Part model, mm, in its own coordinate system. Face numbers are marked on the shaded views. A direction names the side the tool comes from. Round coordinates to 2 decimals unless told otherwise and drop trailing zeros. Write each loop counter-clockwise with the first axis right and the second up, starting at its lowest first coordinate (ties: lowest second). Pieces come first, ordered by that corner, then holes.
from build123d import *

# Parameters (mm, degrees)
FILLET1_R          = 1.3
CHAMFER1_SIZE      = 1
CHAMFER1_SIZE2     = 0.577350269
SKETCH2_OUTSIDE_W  = 37.134
SKETCH2_OUTSIDE_H  = 37.134
CUT_EXTRUDE1_DEPTH = 8
CHAMFER2_SIZE      = 1.6


with BuildPart() as part:
    # Sketch1 → Revolve1 (revolve)
    with BuildSketch(Plane(origin=(0, 0, 0), x_dir=(0, 0, -1), z_dir=(1, 0, 0))):
        Polygon((10, 0), (10, 12), (6.5, 12), (6.5, 14), (12, 14), (12, 8), (13.5, 8), (13.5, 0), align=None)
    revolve(axis=Axis((0, 0, 0), (0, 1, 0)))

    # Fillet1
    fillet1_edges = [part.edges().sort_by_distance(p)[0] for p in [
        (0, 14, 12),
    ]]
    fillet(fillet1_edges, radius=FILLET1_R)

    # Chamfer1
    chamfer1_edges = [part.edges().sort_by_distance(p)[0] for p in [
        (0, 8, 13.5),
    ]]
    chamfer1_side = [part.faces().sort_by_distance(p)[0] for p in [
        (0, 8, 12.381837662),
    ]]
    chamfer(chamfer1_edges, length=CHAMFER1_SIZE, length2=CHAMFER1_SIZE2, reference=chamfer1_side[0])

    # Sketch2 outside → Cut-Extrude1 (cut)
    with BuildSketch(Plane.XZ):
        Rectangle(SKETCH2_OUTSIDE_W, SKETCH2_OUTSIDE_H)
        Polygon((-13.5, 0), (-6.75, -11.691342951), (6.75, -11.691342951), (13.5, 0), (6.75, 11.691342951), (-6.75, 11.691342951), align=None, mode=Mode.SUBTRACT)
    extrude(amount=-CUT_EXTRUDE1_DEPTH, mode=Mode.SUBTRACT)

    # Chamfer2
    chamfer2_edges = [part.edges().sort_by_distance(p)[0] for p in [
        (0, 0, 10),
    ]]
    chamfer(chamfer2_edges, length=CHAMFER2_SIZE)


solid = part.part
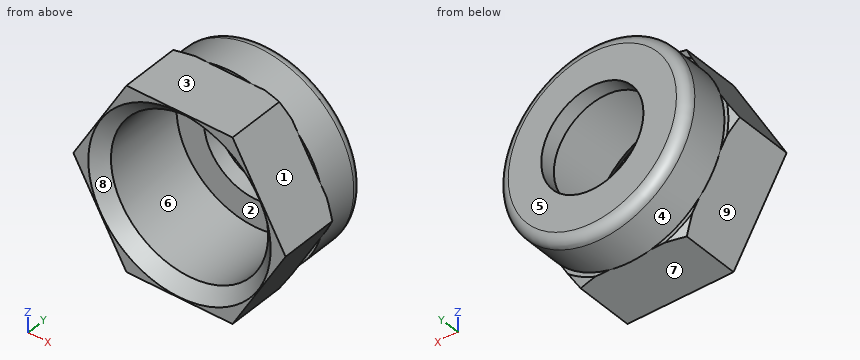
Q1. Saw through at B-B, the plane y = 6. Write the cut outline in (x, z), and give its area (3 significant figures).
Q2. Saw through at D-D, the plane y = 10. Write the cut outline in (x, z).
Q3. Drop flat-ended pins along their axis: P1, Ø0.8, axis at x = 12, z = -0.5, coming from the +Y side; P2, Ø1.5, axis at x = 8.5, y = 8, coming from the +Z side; P3, Ø1, axis at x = 4, y = 7.5, coming from the -Z side. Give the stop position or say it passes through.
Q4. Tool access for the marked faces 1, 2, 3, 4 and 5: list every direction of +Z, -Z, +X, -X, +Y, -Y with a clear straight run to the whole face (end or side of a thin tool).
Q5. Saw through at A-A, the plane x = 0. Write the cut outline in (y, z), and give its area (3 significant figures).
Q6. Saw through at C-C, the plane y = 1.25. Write the cut outline in (x, z), and give its area (3 significant figures).
Q7. Two-plate mould, pull along X, no slides. Class the marked faces 6, 7, 8 and 9: released by +X, released by -X, zero draft, split by the parting line, or undercut.
Q8. Wall check: line 1 (X direction, y = 12.5, z = 0); line 2 (Y direction, x = 5, z = -7); line 3 (Z direction, x = 0, y = 4). Give the ranges that are in metal, low to high.
Computed:
1. outline: (-13.5, 0) - (-6.75, -11.69) - (6.75, -11.69) - (13.5, 0) - (6.75, 11.69) - (-6.75, 11.69) - close; hole circle Ø20 at (0, 0)
1. area: 159 mm2
2. outline: circle Ø24 at (0, 0); hole circle Ø20 at (0, 0)
3. P1: stops at y = 13.63
3. P2: stops at z = 9.95
3. P3: stops at z = -11.69
4. face 1: +Z, +X, -Y
4. face 2: -Y
4. face 3: +Z, +X, -X, -Y
4. face 4: +Y
4. face 5: +Z, -Z, +X, -X, +Y
5. outline: (0, -11.69) - (8, -11.69) - (8, -12) - (12.7, -12) arc R1.3 ccw to (14, -10.7) - (14, -6.5) - (12, -6.5) - (12, -10) - (1.6, -10) - (0, -11.6) - close; (0, 11.6) - (1.6, 10) - (12, 10) - (12, 6.5) - (14, 6.5) - (14, 10.7) arc R1.3 ccw to (12.7, 12) - (8, 12) - (8, 11.69) - (0, 11.69) - close
5. area: 61.8 mm2
6. outline: (-13.5, 0) - (-6.75, -11.69) - (6.75, -11.69) - (13.5, 0) - (6.75, 11.69) - (-6.75, 11.69) - close; hole circle Ø20.7 at (0, 0)
6. area: 137 mm2
7. face 6: undercut
7. face 7: zero draft
7. face 8: undercut
7. face 9: released by -X
8. line 1: x = -12 to -6.5, 6.5 to 12
8. line 2: y = 12 to 14
8. line 3: z = -11.69 to -10, 10 to 11.69
